The model under review builds one solid part; all positions refer to its coordinate system, in mm. A direction names the side the tool comes from. Round coordinates to 2 decimals unless told otherwise and drop trailing zeros. Write each loop counter-clockwise with the first axis right and the second up, starting at its lowest first coordinate (ties: lowest second). Pieces come first, ordered by that corner, then holes. Notation, with made-up numbers: (33.5, 60.5) - (86.5, 60.5) arc R9 ccw to (86.5, 70.5) - close; hole circle Ø1 at (52.5, 50). An arc over 180 degrees is marked (long way). Write each question's results on one line, items separated by ' | '.
```python
from build123d import *

# Parameters (mm, degrees)
F1_DEPTH = 2.5
F2_R     = 0.85
F3_DEPTH = 12.5


with BuildPart() as f1:
    # F0 (on Top) → F1 (new body)
    with BuildSketch(Plane.XY):
        with BuildLine():
            Line((13.081475452, -13.081475452), (1.0606601718, -1.0606601718))
            ThreePointArc((1.0606601718, -1.0606601718), (0, -0.6213203436), (-1.0606601718, -1.0606601718))
            Line((-1.0606601718, -1.0606601718), (-13.081475452, -13.081475452))
            ThreePointArc((-13.081475452, -13.081475452), (-13.5208152802, -14.1421356237), (-13.081475452, -15.2027957955))
            Line((-13.081475452, -15.2027957955), (-1.0606601718, -27.2236110757))
            ThreePointArc((-1.0606601718, -27.2236110757), (0, -27.6629509039), (1.0606601718, -27.2236110757))
            Line((1.0606601718, -27.2236110757), (13.081475452, -15.2027957955))
            ThreePointArc((13.081475452, -15.2027957955), (13.5208152802, -14.1421356237), (13.081475452, -13.081475452))
        make_face()
        with BuildLine():
            Line((-3.8649892248, -12.5063058175), (-4.329398947, -12.5063058175))
            Line((-4.329398947, -12.5063058175), (-6.0112565859, -8.1117745675))
            Line((-6.0112565859, -8.1117745675), (-6.038383322, -8.1117745675))
            add(Edge.make_bspline(
                [(-6.038383322, -8.1117745675), (-5.9906402665, -8.6336929703), (-5.9906402665, -9.353094012)],
                knots=[0, 0, 0, 1, 1, 1], degree=2))
            Line((-5.9906402665, -9.353094012), (-5.9906402665, -12.5063058175))
            Line((-5.9906402665, -12.5063058175), (-6.5234093637, -12.5063058175))
            Line((-6.5234093637, -12.5063058175), (-6.5234093637, -7.5486235258))
            Line((-6.5234093637, -7.5486235258), (-5.6553538082, -7.5486235258))
            Line((-5.6553538082, -7.5486235258), (-4.085258322, -11.638250262))
            Line((-4.085258322, -11.638250262), (-4.0581315859, -11.638250262))
            Line((-4.0581315859, -11.638250262), (-2.4750152665, -7.5486235258))
            Line((-2.4750152665, -7.5486235258), (-1.6134701276, -7.5486235258))
            Line((-1.6134701276, -7.5486235258), (-1.6134701276, -12.5063058175))
            Line((-1.6134701276, -12.5063058175), (-2.1896420026, -12.5063058175))
            Line((-2.1896420026, -12.5063058175), (-2.1896420026, -9.3118613731))
            add(Edge.make_bspline(
                [(-2.1896420026, -9.3118613731), (-2.1896420026, -8.7628162342), (-2.141898947, -8.1182849842)],
                knots=[0, 0, 0, 1, 1, 1], degree=2))
            Line((-2.141898947, -8.1182849842), (-2.1690256832, -8.1182849842))
            Line((-2.1690256832, -8.1182849842), (-3.8649892248, -12.5063058175))
        make_face(mode=Mode.SUBTRACT)
        with BuildLine():
            Line((-8.1334756687, -14.8039748892), (-8.1334756687, -13.4802963582))
            Line((-8.1334756687, -13.4802963582), (-0.6236797201, -13.4802963582))
            Line((-0.6236797201, -13.4802963582), (-0.6236797201, -6.9198086858))
            ThreePointArc((-0.6236797201, -6.9198086858), (-0.9032194318, -6.4583786209), (-0.9135835525, -5.9189782686))
            ThreePointArc((-0.9135835525, -5.9189782686), (0.0168397474, -5.0141534426), (0.9868078824, -5.876451129))
            ThreePointArc((0.9868078824, -5.876451129), (0.9900106564, -6.4384308628), (0.6999988109, -6.9198086858))
            Line((0.6999988109, -6.9198086858), (0.6999988109, -13.4802963582))
            Line((0.6999988109, -13.4802963582), (8.1334756687, -13.4802963582))
            ThreePointArc((8.1334756687, -13.4802963582), (8.5949057336, -13.2007566465), (9.134306086, -13.1903925258))
            ThreePointArc((9.134306086, -13.1903925258), (10.0391309119, -14.1208158258), (9.1768332255, -15.0907839607))
            ThreePointArc((9.1768332255, -15.0907839607), (8.6148534917, -15.0939867347), (8.1334756687, -14.8039748892))
            Line((8.1334756687, -14.8039748892), (0.6999988109, -14.8039748892))
            Line((0.6999988109, -14.8039748892), (0.6999988109, -23.1867600232))
            Line((0.6999988109, -23.1867600232), (-0.6236797201, -23.1867600232))
            Line((-0.6236797201, -23.1867600232), (-0.6236797201, -14.8039748892))
            Line((-0.6236797201, -14.8039748892), (-8.1334756687, -14.8039748892))
        make_face(mode=Mode.SUBTRACT)
        with BuildLine():
            Line((2.2484090003, -12.5063053519), (2.2484090003, -7.5486230602))
            Line((2.2484090003, -7.5486230602), (3.6492336531, -7.5486230602))
            add(Edge.make_bspline(
                [(3.6492336531, -7.5486230602), (4.6355617781, -7.5486230602), (5.0766425073, -7.8437619491)],
                knots=[0, 0, 0, 1, 1, 1], degree=2))
            add(Edge.make_bspline(
                [(5.0766425073, -7.8437619491), (5.5177232364, -8.138900838), (5.5177232364, -8.7758366019)],
                knots=[0, 0, 0, 1, 1, 1], degree=2))
            add(Edge.make_bspline(
                [(5.5177232364, -8.7758366019), (5.5177232364, -9.2174598657), (5.2719550073, -9.5039181991)],
                knots=[0, 0, 0, 1, 1, 1], degree=2))
            add(Edge.make_bspline(
                [(5.2719550073, -9.5039181991), (5.0261867781, -9.7903765324), (4.5541815698, -9.8750119491)],
                knots=[0, 0, 0, 1, 1, 1], degree=2))
            Line((4.5541815698, -9.8750119491), (4.5541815698, -9.9086491019))
            add(Edge.make_bspline(
                [(4.5541815698, -9.9086491019), (5.6837388614, -10.101791463), (5.6837388614, -11.0957150741)],
                knots=[0, 0, 0, 1, 1, 1], degree=2))
            add(Edge.make_bspline(
                [(5.6837388614, -11.0957150741), (5.6837388614, -11.7597775741), (5.2345201114, -12.133041463)],
                knots=[0, 0, 0, 1, 1, 1], degree=2))
            add(Edge.make_bspline(
                [(5.2345201114, -12.133041463), (4.7853013614, -12.5063053519), (3.9780096948, -12.5063053519)],
                knots=[0, 0, 0, 1, 1, 1], degree=2))
            Line((3.9780096948, -12.5063053519), (2.2484090003, -12.5063053519))
        make_face(mode=Mode.SUBTRACT)
    extrude(amount=F1_DEPTH)

    # F2 (on Right) → F3 (cut, symmetric)
    with BuildSketch(Plane.YZ):
        with Locations((-2.4908210296, 1.292226194)):
            Circle(F2_R)
    extrude(amount=F3_DEPTH, both=True, mode=Mode.SUBTRACT)


solid = f1.part
```
Q1. Insertion check: P1, Ø0.8, axis at y = -11.5, z = 1, coming from the -X side; P2, Ø0.8, axis at y = -10, z = 1, coming from the -X side; P3, Ø0.8, axis at x = -4.5, z = 1.5, coming from the -Y side. Each pin has a flat end and moves straight along its axis. Give the tip position at first contact, or say it passes through.
Evaluation:
P1: stops at x = -11.9 | P2: stops at x = -10.4 | P3: stops at y = -24.18
Q2. We need section B-B (x = -7.75). State the section outline as (y, z) points.
Evaluation:
outline: (-20.53, 0) - (-14.8, 0) - (-14.8, 2.5) - (-20.53, 2.5) - close; (-13.48, 0) - (-7.75, 0) - (-7.75, 2.5) - (-13.48, 2.5) - close
Q3. We need section A-A (y = -16.75). State the section outline as (x, z) points, plus the area to 3 significant figures.
Evaluation:
outline: (-11.53, 0) - (-0.62, 0) - (-0.62, 2.5) - (-11.53, 2.5) - close; (0.7, 0) - (11.53, 0) - (11.53, 2.5) - (0.7, 2.5) - close | area: 54.4 mm^2
Q4. For probe 1 along Y at (x, z) = (2.5, 1.1); probe 2 along Y at (x, z) = (0, 1.85); probe 3 along Y at (x, z) = (1.5, 0.2), list the stretches that pass through material, from the lowest coordinate up.
Evaluation:
probe 1: y = -25.78 to -14.8, -13.48 to -12.51, -7.55 to -3.32 | probe 2: y = -27.66 to -23.19, -5.01 to -3.13, -1.85 to -0.62 | probe 3: y = -26.78 to -14.8, -13.48 to -1.5
Q5. We need section D-D (y = -3.75). State the section outline as (x, z) points.
Evaluation:
outline: (-3.75, 0) - (3.75, 0) - (3.75, 2.5) - (-3.75, 2.5) - close
Q6. The part is to be moulded in two halves that separate along Y. For faces 3 (the flat face through (-7.155, -21.129, 1.232)), 4 (the cylindrical face through (-0.9, -6.47, 1.23)), 5 (the flat face through (1, -15, 2.5)), say which applies: released by +Y, released by -Y, zero draft, split by the parting line, or undercut.
Evaluation:
face 3: released by -Y | face 4: undercut | face 5: zero draft
Q7. Tool access review of faces 1 (the flat face through (-7, -7, 1)), 2 (the flat face through (-4, -13.48, 1)): name each direction out of +Z, -Z, +X, -X, +Y, -Y from which nothing blocks a thin tool from reaching the whole face with its end or side.
Evaluation:
face 1: +Z, -Z, -X, +Y | face 2: +Z, -Z
Q8. We need section C-C (z = 0.9). State how many separate pieces and enclosed holes the cut face has, plus the area to 3 significant figures.
Evaluation:
separate pieces: 2 | enclosed holes: 3 | area: 317 mm^2
